Check sheet for the modelled part. Datum: model origin and axes. Units: mm. A direction names the side the tool comes from. Give positions to 0.01 mm unless a question says otherwise; leave off trailing zeros. Order: outer loops, then holes, each group sorted by start corner. A loop starts at its lowest first (then second) coordinate and runs counter-clockwise, first axis right, second up.
Item 1: Sectioned sample at C-C on x = 30. Record the boundary of the cut face in (y, z).
Item 2: Sectioned sample at D-D on x = 36.5. Record the boundary of the cut face in (y, z).
Item 3: Material ranges on line 1 along Y through (x, z) = (35, 1.1); line 2 along Y through (x, z) = (47, 1.25); line 3 along X through (y, z) = (0.1, 0.5), recorded low to high.
Item 4: Release check for a two-part mould opening along Y. For faces 4 (the flat face through (23, 0, 0)), 5 (the cylindrical face through (0, 1, 1)), 6 (the flat face through (32.5, -1.5, 0.7)) record: released by +Y, released by -Y, zero draft, split by the parting line, or undercut.
Item 5: Sectioned sample at B-B on x = 0. Record the boundary of the cut face in (y, z).
Item 6: Sectioned sample at A-A on z = 1. Record the boundary of the cut face in (x, y).
Item 7: Access from +Z, -Z, +X, -X, +Y, -Y to the whole of each face (thin tool, end or side, straight path). Record for faces 1 (the flat face through (41, 1.5, 1)), 2 (the flat face through (41, -1.5, 1)), 3 (the flat face through (23, 0, 1.5)).
Item 8: Gauge pin test, flat ends, axial feed: P1, Ø1.2, axis at x = 47, y = 0, coming from the +Z side; P2, Ø0.6, axis at x = 32.5, z = 0.5, coming from the +Y side. Record the tip position at first contact, or that the pin passes through.
Autodesk Inventor part; units mm, degrees
ref_plane "YZ Plane" through (0, 0, 0) normal (1, 0, 0) x (0, 1, 0)
ref_plane "XZ Plane" through (0, 0, 0) normal (0, 1, 0) x (-1, 0, 0)
ref_plane "XY Plane" through (0, 0, 0) normal (0, 0, 1) x (1, 0, 0)
sketch "Sketch1" plane through (0, 0, 0) normal (0, 0, 1) x (1, 0, 0)
  circle A0 centre (0, 0) radius 1
  circle A1 centre (0, 0) radius 2
  line L0 (0, 0) -> (47, 0) construction
  circle A2 centre (47, 0) radius 2
  circle A3 centre (47, 0) radius 1
  line L1 (1, 1.5) -> (46, 1.5)
  line L2 (46, 1.5) -> (46, -1.5)
  line L3 (46, -1.5) -> (1, -1.5)
  line L4 (1, -1.5) -> (1, 1.5)
  line L5 (1, 1.5) -> (46, -1.5) construction
  line L6 (46, 1.5) -> (1, -1.5) construction
  point P0 (23.5, 0)
  point P1 (1.3229, -1.5)
  point P2 (45.6771, -1.5)
  point P3 (45.6771, 1.5)
  point P4 (1.3229, 1.5)
  dimension "d0" = 2
  dimension "d1" = 4
  dimension "d8" = 3
  dimension "d9" = 47
extrude "Extrusion1" add sketch "Sketch1" along normal blind 1.5
fillet "Fillet2" radius 2 4 edges at (1.3229, 1.5, 0.75) (45.6771, 1.5, 0.75) (45.6771, -1.5, 0.75) (1.3229, -1.5, 0.75)
sketch "Sketch3" plane through (0, 0, 1.5) normal (0, 0, 1) x (1, 0, 0)
  line L0 (-12.2, 0) -> (59.2, 0)
  circle A0 centre (35, 0) radius 0.75
  circle A1 centre (30, 0) radius 0.75
  circle A2 centre (47, 0) radius 1
  point P0 (0, 0)
  dimension "d11" = 12
  dimension "d12" = 5
  dimension "d13" = 1.5
extrude "Extrusion2" cut sketch "Sketch3" against normal through all contours A1 L0 | A0 L0 | L0 A0 | L0 A1
sketch "Sketch4" plane through (0, 0, 1.5) normal (0, 0, 1) x (1, 0, 0)
  circle A0 centre (30, 0) radius 0.75
  circle A1 centre (30, 0) radius 2
  circle A2 centre (35, 0) radius 0.75
  circle A3 centre (35, 0) radius 2
  point P0 (0, 0)
  dimension "d16" = 4
extrude "Extrusion3" add sketch "Sketch4" against normal up to surface (1.5 mm away)
fillet "Fillet3" radius 2 8 edges at (28.6771, 1.5, 0.75) (31.3229, 1.5, 0.75) (33.6771, 1.5, 0.75) (36.3229, 1.5, 0.75) (33.6771, -1.5, 0.75) (36.3229, -1.5, 0.75) (28.6771, -1.5, 0.75) (31.3229, -1.5, 0.75)
properties part number "ff"
Report:
1. outline: (-2, 0) - (-0.75, 0) - (-0.75, 1.5) - (-2, 1.5) - close; (0.75, 0) - (2, 0) - (2, 1.5) - (0.75, 1.5) - close
2. outline: (-1.55, 0) - (1.55, 0) - (1.55, 1.5) - (-1.55, 1.5) - close
3. line 1: y = -2 to -0.75, 0.75 to 2
3. line 2: y = -2 to -1, 1 to 2
3. line 3: x = -2 to -0.99, 0.99 to 29.26, 30.74 to 34.26, 35.74 to 46.01, 47.99 to 49
4. face 4: zero draft
4. face 5: undercut
4. face 6: released by -Y
5. outline: (-2, 0) - (-1, 0) - (-1, 1.5) - (-2, 1.5) - close; (1, 0) - (2, 0) - (2, 1.5) - (1, 1.5) - close
6. outline: (0.97, -1.75) arc R2 cw to (1.94, -1.5) - (28.06, -1.5) arc R2 cw to (29.03, -1.75) arc R2 ccw to (30.97, -1.75) arc R2 cw to (31.94, -1.5) - (33.06, -1.5) arc R2 cw to (34.03, -1.75) arc R2 ccw to (35.97, -1.75) arc R2 cw to (36.94, -1.5) - (45.06, -1.5) arc R2 cw to (46.03, -1.75) arc R2 ccw (long way) to (46.03, 1.75) arc R2 cw to (45.06, 1.5) - (36.94, 1.5) arc R2 cw to (35.97, 1.75) arc R2 ccw to (34.03, 1.75) arc R2 cw to (33.06, 1.5) - (31.94, 1.5) arc R2 cw to (30.97, 1.75) arc R2 ccw to (29.03, 1.75) arc R2 cw to (28.06, 1.5) - (1.94, 1.5) arc R2 cw to (0.97, 1.75) arc R2 ccw (long way) to start; hole circle Ø2 at (0, 0); hole circle Ø1.5 at (30, 0); hole circle Ø1.5 at (35, 0); hole circle Ø2 at (47, 0)
7. face 1: +Z, -Z, +Y
7. face 2: +Z, -Z, -Y
7. face 3: +Z, +X, -X, +Y, -Y
8. P1: passes through
8. P2: stops at y = 1.5
